Source: CAD feature listing. Evaluate the final solid. Frame: model axes, mm. A direction names the side the tool comes from. Give positions to 0.01 mm unless a question says otherwise; leave off trailing zeros. Write each loop counter-clockwise with the first axis right and the second up, starting at its lowest first coordinate (ties: lowest second). Pieces come first, ordered by that corner, then holes. Notation, with made-up numbers: (61, 17) -> (66, 17) arc R31 cw to (66, 45) -> close; hole circle Ø5 at (81.5, -29). An arc over 180 degrees is marked (long way). Use one line per item in the form item = value. Start each with the question number.
(1) Cut plane A-A, the plane z = -13.5. Output: boundary loops of the cut face in (x, y).
(2) Set-up query: faces 1 (the face through (1.2, -1.2, 0)), 2 (the face through (-1.495, 0.88, 2.014)), 3 (the face through (0, 2, 3)). Return all of +Z, -Z, +X, -X, +Y, -Y with unobstructed straight access to the full face (end or side cutting, diameter ignored); none if empty.
(3) First-contact query: P1, Ø1.5, axis at x = 0, y = -0.5, coming from the +Z side; P2, Ø1, axis at y = -1.5, z = -16, coming from the -X side; P3, Ø1, axis at x = 0, z = -13, coming from the +Y side. Flat tips, straight axial feed; report the tip coordinate or a pass-through.
(4) Material intervals for line 1 along Y through (x, z) = (1.8, 1.5); line 2 along Z through (x, y) = (1.6, 1.2); line 3 along X through (y, z) = (0.1, 1.5), sorted ascending. Write a range as from..to.
(5) Draft query along X for faces 4 (the face through (-1.509, -0.855, 2.014)), 5 (the face through (0, 0, -20)), 6 (the face through (1.509, 0.855, 2.014)), 7 (the face through (2.62, 0.82, 1.23)). Return one class per face: pulls with the +X half, pulls with the -X half, needs draft (parallel to the pull), parting line crosses it, or undercut.
from build123d import *

# Parameters (mm, degrees)
SKETCH1_R          = 1.5
EXTRUDE1_DEPTH     = 20
SKETCH2_R          = 2.745016825
EXTRUDE2_DEPTH     = 3
CUT_EXTRUDE1_DEPTH = 2
FILLET1_R          = 0.5
FILLET2_R          = 1


with BuildPart() as part:
    # Sketch1 → Extrude1 (new body)
    with BuildSketch(Plane.XY):
        Circle(SKETCH1_R)
    extrude(amount=-EXTRUDE1_DEPTH)

    # Sketch2 → Extrude2 (add)
    with BuildSketch(Plane.XY):
        Circle(SKETCH2_R)
    extrude(amount=EXTRUDE2_DEPTH)

    # Sketch3 → Cut-Extrude1 (cut)
    with BuildSketch(Plane.XY.offset(3)):
        Polygon((-2.003123501, 0), (-1.00156175, -1.734755838), (1.00156175, -1.734755838), (2.003123501, 0), (1.00156175, 1.734755838), (-1.00156175, 1.734755838), align=None)
    extrude(amount=-CUT_EXTRUDE1_DEPTH, mode=Mode.SUBTRACT)

    # Fillet1
    fillet1_edges = [part.edges().sort_by_distance(p)[0] for p in [
        (-2.745016825, 0, 3),
    ]]
    fillet(fillet1_edges, radius=FILLET1_R)

    # Fillet2
    fillet2_edges = [part.edges().sort_by_distance(p)[0] for p in [
        (-1.5, 0, -20),
    ]]
    fillet(fillet2_edges, radius=FILLET2_R)


solid = part.part
Geometry says:
q1.outline = circle Ø3 at (0, 0)
q2.face_1 = -Z
q2.face_2 = +Z
q2.face_3 = +Z, +X, -X, +Y, -Y
q3.P1 = 1
q3.P2 = -1.12
q3.P3 = 1.5
q4.line_1 = -2.07..-0.35, 0.35..2.07
q4.line_2 = 0..3
q4.line_3 = -2.74..-1.95, 1.95..2.74
q5.face_4 = undercut
q5.face_5 = needs draft
q5.face_6 = undercut
q5.face_7 = parting line crosses it
